Geometry check sheet. Reference: the model listing, model coordinates, mm. A direction names the side the tool comes from. Coordinates: 2 decimals unless noted, no trailing zeros. Loops run counter-clockwise (first coordinate to the right, second up) from the corner with the lowest first, then second, coordinate; pieces in that order, holes last. Notation, with made-up numbers: (33.5, 87) - (47.5, 87) arc R8 ccw to (47.5, 101) - close; hole circle Ø7 at (52.25, 17.25). An arc over 180 degrees is marked (long way). Write each question's results on one line, items separated by ' | '. Start each with the question number.
(1) Sectioned sample at A-A (x = 0). Enter the section's corners in (y, z) (1 decimal), plus the area to 3 significant figures.
(2) Access from +Z, -Z, +X, -X, +Y, -Y to the whole of each face (thin tool, end or side, straight path). Record for faces 1 (the face through (-2.57, 4.32, -1.64)), 2 (the face through (0.2, 0, 3.2)), 3 (the face through (-0.2, 0, -3.2)).
(3) Material ranges on probe 1 along Y at (x, z) = (2.25, 2.5); probe 2 along Z at (x, y) = (-2.5, 8.25); probe 3 along X at (y, z) = (3.25, 2.25), recorded low to high.
(4) Sectioned sample at C-C (z = 3.5). Enter the section's corners in (x, y).
(5) Sectioned sample at B-B (y = 2.5). Enter the section's corners in (x, z), plus the area to 3 significant figures.
(6) Go/stop test with flat-tipped pins: pin 1 Ø3 at (y, z) = (4.5, -2.5) entering from +X; pin 2 Ø1 at (x, z) = (1.5, -2) entering from +Y (3 decimals). Record where each tip stops, or that it passes through.
from build123d import *

# Parameters (mm, degrees)
SKETCH1_R           = 3.048
BOSS_EXTRUDE1_DEPTH = 9.525
CHAMFER1_SIZE       = 0.762
SKETCH2_R           = 3.81
BOSS_EXTRUDE2_DEPTH = 1.5875
SKETCH4_W           = 5.15979919
SKETCH4_H           = 9.269210688
SKETCH4_W_2         = 9.619339919
SKETCH4_H_2         = 8.458385102
CUT_EXTRUDE1_DEPTH  = 11.943391842


with BuildPart() as part:
    # Sketch1 → Boss-Extrude1 (new body)
    with BuildSketch(Plane(origin=(0, 0, 0), x_dir=(1, 0, 0), z_dir=(0, 1, 0))):
        with Locations(Location((0, 0, 0), (0, 0, 90))):
            Circle(SKETCH1_R)
    extrude(amount=BOSS_EXTRUDE1_DEPTH)

    # Chamfer1
    chamfer1_edges = [part.edges().sort_by_distance(p)[0] for p in [
        (0, 9.525, 3.048),
    ]]
    chamfer(chamfer1_edges, length=CHAMFER1_SIZE)

    # Sketch2 → Boss-Extrude2 (add)
    with BuildSketch(Plane.XZ):
        with Locations(Location((0, 0, 0), (0, 0, 270))):
            Circle(SKETCH2_R)
    extrude(amount=BOSS_EXTRUDE2_DEPTH)

    # Sketch4 → Cut-Extrude1 (cut, through all)
    with BuildSketch(Plane(origin=(0, 0, 0), x_dir=(1, 0, 0), z_dir=(0, 1, 0))):
        with Locations((-5.627899595, 0)):
            Rectangle(SKETCH4_W, SKETCH4_H)
        with Locations((7.85766996, 0)):
            Rectangle(SKETCH4_W_2, SKETCH4_H_2)
    extrude(amount=-CUT_EXTRUDE1_DEPTH, mode=Mode.SUBTRACT)


solid = part.part
Outcome:
1) outline: (-1.6, -3.8) - (0, -3.8) - (0, -3) - (8.8, -3) - (9.5, -2.3) - (9.5, 2.3) - (8.8, 3) - (0, 3) - (0, 3.8) - (-1.6, 3.8) - close | area: 69.6 mm2
2) face 1: +Y | face 2: +Z, +Y | face 3: -Z, +Y
3) probe 1: y = -1.59 to 0 | probe 2: z = -1.74 to 1.74 | probe 3: x = -2.06 to 2.06
4) outline: (-1.51, -1.59) - (1.51, -1.59) - (1.51, 0) - (-1.51, 0) - close
5) outline: circle Ø6.1 at (0, 0) | area: 29.2 mm2
6) pin 1: stops at x = 2.88 | pin 2: stops at y = 9.525
